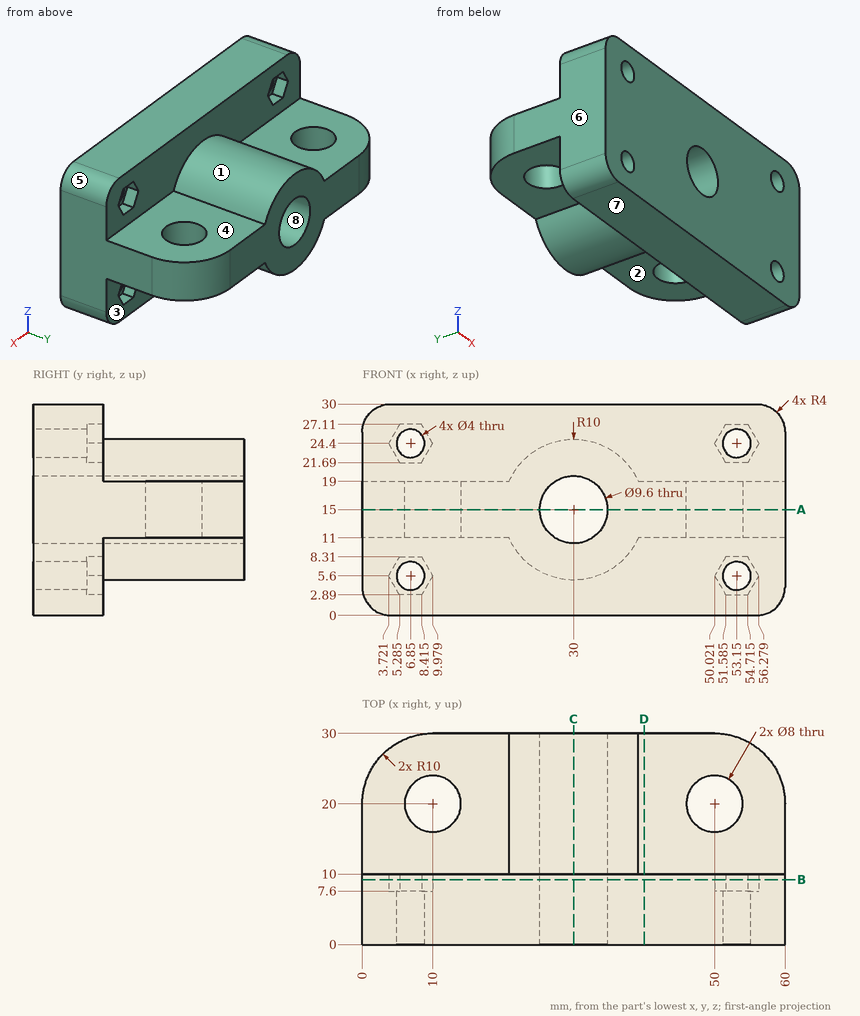
Answer from the drawing. Dimensions are ordinates in mm from the lowest x, y and z of the part. A direction names the side the tool comes from. Give positions to 0.01 mm unless a question says otherwise; leave off trailing zeros. Loops run counter-clockwise (first coordinate to the right, second up) from the corner with the lowest first, then second, coordinate; pieces in that order, holes last. Notation, with made-up numbers: (-28, 3.25) -> (26, 3.25) arc R13 cw to (26, 22.25) -> close; hole circle Ø8 at (9.25, 4.5). An arc over 180 degrees is marked (long way). Use a Markdown table: item, result.
Q1. Each of these flat-tipped pins is pushed along its axis until it touches: pin 1 (1.5 mm diameter, centred on x = 13, y = 16.5, fed in from +Z); pin 2 (1 mm diameter, centred on x = 47, z = 5, fed in from +Y); pin 3 (6.5 mm diameter, centred on x = 10, y = 20, fed in from +Z); pin 4 (6 mm diameter, centred on x = 32.5, y = 18.5, fed in from +Z). Where does it stop, or does it pass through?
Solved:
| item | result |
|---|---|
| pin 1 | stops at z = 19 |
| pin 2 | stops at y = 10 |
| pin 3 | passes through |
| pin 4 | stops at z = 25 |
Q2. Find the intervals of material crossed by line 1 along Z through (x, y) = (6.85, 2.75); line 2 along X through (y, z) = (14, 15); line 3 along X through (y, z) = (20.25, 13.5), in increasing order.
Solved:
| item | result |
|---|---|
| line 1 | z = 0 to 3.6, 7.6 to 22.4, 26.4 to 30 |
| line 2 | x = 0 to 25.2, 34.8 to 60 |
| line 3 | x = 0 to 6.01, 13.99 to 25.44, 34.56 to 46.01, 53.99 to 60 |
Q3. Determine the mould class of the marked faces 5, 6, 7 and 8 for opening direction X: pulls with the +X half, pulls with the -X half, needs draft (parallel to the pull), parting line crosses it, or undercut.
Solved:
| item | result |
|---|---|
| face 5 | pulls with the +X half |
| face 6 | pulls with the -X half |
| face 7 | needs draft |
| face 8 | undercut |
Q4. Section A-A, the plane z = 15 is taken. Determine the outline of the cut face in (x, y).
Solved:
| item | result |
|---|---|
| outline | (0, 0) -> (25.2, 0) -> (25.2, 30) -> (10, 30) arc R10 ccw to (0, 20) -> close; (34.8, 0) -> (60, 0) -> (60, 20) arc R10 ccw to (50, 30) -> (34.8, 30) -> close; hole circle Ø8 at (10, 20); hole circle Ø8 at (50, 20) |
Q5. Section D-D, the plane x = 40 is taken. Determine the outline of the cut face in (y, z), then the cut area to 3 significant figures.
Solved:
| item | result |
|---|---|
| outline | (0, 0) -> (10, 0) -> (10, 11) -> (30, 11) -> (30, 19) -> (10, 19) -> (10, 30) -> (0, 30) -> close |
| area | 460 mm^2 |
Q6. Section C-C, the plane x = 30 is taken. Determine the outline of the cut face in (y, z).
Solved:
| item | result |
|---|---|
| outline | (0, 0) -> (10, 0) -> (10, 5) -> (30, 5) -> (30, 10.2) -> (0, 10.2) -> close; (0, 19.8) -> (30, 19.8) -> (30, 25) -> (10, 25) -> (10, 30) -> (0, 30) -> close |
Q7. Section B-B, the plane y = 9.25 is taken. Count the separate pieces of the cut face and the enclosed holes in it, then the cut area to 3 significant figures.
Solved:
| item | result |
|---|---|
| separate pieces | 1 |
| enclosed holes | 5 |
| area | 1,610 mm^2 |
Q8. A tool of negligible diameter and unlimited length cuts with its end or side. For the marked faces 1, 2, 3 and 4, from which of +Z, -Z, +X, -X, +Y, -Y can it reach the whole face along a straight path? Write none if from no direction.
Solved:
| item | result |
|---|---|
| face 1 | +Z, +Y |
| face 2 | -Z, +X, +Y |
| face 3 | -Z, +Y |
| face 4 | +Z, +X, +Y |
